from build123d import *

# Parameters (mm, degrees)
F0_W     = 78.74
F0_H     = 63.5
F1_DEPTH = 35.56
F2_W     = 15.24
F2_H     = 63.5
F3_DEPTH = 127
F4_R     = 5.08
F5_DEPTH = 76.2


with BuildPart() as f1:
    # F0 (on Front) → F1 (new body)
    with BuildSketch(Plane.XZ):
        Polygon((-57.15, 7.366), (-57.15, 0), (57.15, 0), (57.15, 7.366), (39.37, 7.366), (-39.37, 7.366), align=None)
        with Locations((0, 39.116)):
            Rectangle(F0_W, F0_H)
    extrude(amount=F1_DEPTH)

    # F2 (on face) → F3 (cut)
    with BuildSketch(Plane.YZ.offset(39.37)):
        with Locations((-17.78, 39.116)):
            Rectangle(F2_W, F2_H)
    extrude(amount=-F3_DEPTH, mode=Mode.SUBTRACT)

    # F4 (on face) → F5 (cut)
    with BuildSketch(Plane.XZ.offset(35.56)):
        with Locations((0, 39.116)):
            Circle(F4_R)
    extrude(amount=-F5_DEPTH, mode=Mode.SUBTRACT)


solid = f1.part
Could you check a few things on this model? Use its own coordinates, in mm. A direction names the side the tool comes from. Give positions to 0.01 mm unless a question says otherwise; leave off trailing zeros. Write each loop counter-clockwise with the first axis right and the second up, starting at its lowest first coordinate (ties: lowest second). Pieces come first, ordered by that corner, then holes. Notation, with made-up numbers: (-25.5, 18) - (11.5, 18) arc R29 ccw to (11.5, 50) - close; hole circle Ø9 at (46.25, -25). An arc over 180 degrees is marked (long way). Use CSV: the item, a comma, the result in double quotes. Start each with the question number.
Item 1: I'm going to push flat-ended pins straight in: pin 1 (18 mm diameter, centred on x = 4.5, y = -16, fed in from +Z); pin 2 (8 mm diameter, centred on y = -4, z = 46.5, fed in from -X); pin 3 (5 mm diameter, centred on y = -29, z = 30.5, fed in from +X); pin 4 (2 mm diameter, centred on x = 2.5, y = -19.5, fed in from +Z). Where does each tip first touch, or does it pass through?
Item 2: For faces 1 (the face through (-39.37, -5, 39)), 2 (the face through (39.37, -30, 39)), 3 (the face through (-1, -18, 0)), 4 (the face through (4.845, -30.551, 40.642)), 5 (the face through (1, -10.16, 32)), which set-ups out of +Z, -Z, +X, -X, +Y, -Y let a thin tool reach every point of the face, with its end or its side?
Item 3: If we mould it in two halves opening along Y, with no side actions, what happens to faces 6 (the face through (1, -25.4, 32)), 7 (the face through (-1, -5, 70.866)), 8 (the face through (1, -18, 7.366)), 9 (the face through (-1, -35.56, 28))? For each: pulls with the +Y half, pulls with the -Y half, needs draft (parallel to the pull), parting line crosses it, or undercut.
Item 4: I want a section at A-A, the plane x = 0. Please give me the cut outline in (y, z), then the cut area to 3 significant figures.
Item 5: I want a section at D-D, the plane x = 45.5. Please give me the cut outline in (y, z), then the cut area to 3 significant figures.
Item 6: I want a section at C-C, the plane y = -8.5. Please give me the cut outline in (x, z).
Item 7: If I drill on line 1 along Y through (x, z) = (4, 19); line 2 along Z through (x, y) = (0, -32); line 3 along X through (y, z) = (-2, 30), over which ranges is the centre line in solid material (lowest first)?
Item 8: I want a section at B-B, the plane z = 48. Please give me the cut outline in (x, y), then the cut area to 3 significant figures.
Findings:
1,pin 1,"stops at z = 70.87"
1,pin 2,"stops at x = -39.37"
1,pin 3,"stops at x = 39.37"
1,pin 4,"stops at z = 7.37"
2,face 1,"+Z, -X, +Y, -Y"
2,face 2,"+Z, +X, +Y, -Y"
2,face 3,"-Z, +X, -X, +Y, -Y"
2,face 4,"+Y, -Y"
2,face 5,"+Z, +X, -X"
3,face 6,"undercut"
3,face 7,"needs draft"
3,face 8,"undercut"
3,face 9,"pulls with the -Y half"
4,outline,"(-35.56, 0) - (0, 0) - (0, 34.04) - (-10.16, 34.04) - (-10.16, 7.37) - (-25.4, 7.37) - (-25.4, 34.04) - (-35.56, 34.04) - close; (-35.56, 44.2) - (-25.4, 44.2) - (-25.4, 70.87) - (-35.56, 70.87) - close; (-10.16, 44.2) - (0, 44.2) - (0, 70.87) - (-10.16, 70.87) - close"
4,area,"1,350 mm2"
5,outline,"(-35.56, 0) - (0, 0) - (0, 7.37) - (-35.56, 7.37) - close"
5,area,"262 mm2"
6,outline,"(-57.15, 0) - (57.15, 0) - (57.15, 7.37) - (39.37, 7.37) - (39.37, 70.87) - (-39.37, 70.87) - (-39.37, 7.37) - (-57.15, 7.37) - close; hole circle Ø10.16 at (0, 39.12)"
7,line 1,"y = -35.56 to -25.4, -10.16 to 0"
7,line 2,"z = 0 to 34.04, 44.2 to 70.87"
7,line 3,"x = -39.37 to 39.37"
8,outline,"(-39.37, -35.56) - (39.37, -35.56) - (39.37, -25.4) - (-39.37, -25.4) - close; (-39.37, -10.16) - (39.37, -10.16) - (39.37, 0) - (-39.37, 0) - close"
8,area,"1,600 mm2"
